Could you check a few things on this model? Use its own coordinates, in mm. A direction names the side the tool comes from. Round coordinates to 2 decimals unless told otherwise and drop trailing zeros. Write each loop counter-clockwise with the first axis right and the second up, starting at its lowest first coordinate (ties: lowest second). Pieces come first, ordered by that corner, then holes. Notation, with made-up numbers: (53, -10) -> (93, -10) arc R10 ccw to (93, 4) -> close; hole circle Ø3 at (-32.75, 79.5). An arc over 180 degrees is marked (long way). Return JSON: item names as keys, results as strings.
from build123d import *

# Parameters (mm, degrees)
SKETCH1_W           = 15
SKETCH1_H           = 10
BOSS_EXTRUDE1_DEPTH = 60
SKETCH2_W           = 15
SKETCH2_H           = 3
BOSS_EXTRUDE2_DEPTH = 10
SKETCH3_W           = 11
SKETCH3_H           = 18.791084145
CUT_EXTRUDE1_DEPTH  = 71.700070721
FILLET1_R           = 1
CUT_EXTRUDE2_DEPTH  = 72.107313267


with BuildPart() as part:
    # Sketch1 → Boss-Extrude1 (new body)
    with BuildSketch(Plane(origin=(0, 0, 0), x_dir=(1, 0, 0), z_dir=(0, 1, 0))):
        Rectangle(SKETCH1_W, SKETCH1_H)
    extrude(amount=BOSS_EXTRUDE1_DEPTH)

    # Sketch2 → Boss-Extrude2 (add)
    with BuildSketch(Plane(origin=(0, 60, 0), x_dir=(1, 0, 0), z_dir=(0, 1, 0))):
        Rectangle(SKETCH2_W, SKETCH2_H)
    extrude(amount=BOSS_EXTRUDE2_DEPTH)

    # Sketch3 → Cut-Extrude1 (cut, through all)
    with BuildSketch(Plane.XY.offset(1.5)):
        with Locations((0, 70.395542073)):
            Rectangle(SKETCH3_W, SKETCH3_H)
    extrude(amount=-CUT_EXTRUDE1_DEPTH, mode=Mode.SUBTRACT)

    # Fillet1
    fillet1_edges = [part.edges().sort_by_distance(p)[0] for p in [
        (-5.5, 70, 0),
        (5.5, 70, 0),
        (5.5, 61, 0),
        (-5.5, 61, 0),
        (-7.5, 70, 0),
        (7.5, 70, 0),
    ]]
    fillet(fillet1_edges, radius=FILLET1_R - 0.0001)  # a hair under: the kernel refuses the full size

    # Sketch4 → Cut-Extrude2 (cut, through all)
    with BuildSketch(Plane.XY.offset(5)):
        with BuildLine():
            Line((-1.5, 5), (1.5, 5))
            ThreePointArc((1.5, 5), (3.621320344, 5.878679656), (4.5, 8))
            Line((4.5, 8), (4.5, 52))
            ThreePointArc((4.5, 52), (3.621320344, 54.121320344), (1.5, 55))
            Line((1.5, 55), (-1.5, 55))
            ThreePointArc((-1.5, 55), (-3.621320344, 54.121320344), (-4.5, 52))
            Line((-4.5, 52), (-4.5, 8))
            ThreePointArc((-4.5, 8), (-3.621320344, 5.878679656), (-1.5, 5))
        make_face()
    extrude(amount=-CUT_EXTRUDE2_DEPTH, mode=Mode.SUBTRACT)


solid = part.part
1) I want a section at D-D, the plane x = -3.5. Please give me the cut outline in (y, z), and give its area (3 significant figures).
Return value:
{"outline": "(0, -5) -> (5.76, -5) -> (5.76, 5) -> (0, 5) -> close; (54.24, -5) -> (60, -5) -> (60, -1.5) -> (61, -1.5) -> (61, 1.5) -> (60, 1.5) -> (60, 5) -> (54.24, 5) -> close", "area": "118 mm²"}
2) I want a section at C-C, the plane z = -3. Please give me the cut outline in (x, y).
Return value:
{"outline": "(-7.5, 0) -> (7.5, 0) -> (7.5, 60) -> (-7.5, 60) -> close; hole (-4.5, 8) arc R3 ccw to (-1.5, 5) -> (1.5, 5) arc R3 ccw to (4.5, 8) -> (4.5, 52) arc R3 ccw to (1.5, 55) -> (-1.5, 55) arc R3 ccw to (-4.5, 52) -> close"}
3) I want a section at A-A, the plane y = 10.5. Please give me the cut outline in (x, z).
Return value:
{"outline": "(-7.5, -5) -> (-4.5, -5) -> (-4.5, 5) -> (-7.5, 5) -> close; (4.5, -5) -> (7.5, -5) -> (7.5, 5) -> (4.5, 5) -> close"}
4) If I drill on probe 1 along X at (y, z) = (37.5, 2); probe 2 along Y at (x, z) = (-1.5, -1); probe 3 along Y at (x, z) = (-7, -4.5), over which ranges is the centre line in solid material (lowest first)? Write a range as [from, to].
Return value:
{"probe 1": "[-7.5, -4.5], [4.5, 7.5]", "probe 2": "[0, 5], [55, 61]", "probe 3": "[0, 60]"}
5) For faces 1 (the face through (-7.5, 34, 0)), 2 (the face through (0, 55, 0)), 3 (the face through (0, 60, -3)), 4 (the face through (0, 60.2, 1.5)), 5 (the face through (5.5, 65, 0)), which set-ups out of +Z, -Z, +X, -X, +Y, -Y let a thin tool reach every point of the face, with its end or its side?
Return value:
{"face 1": "+Z, -Z, -X, +Y, -Y", "face 2": "+Z, -Z", "face 3": "-Z, +X, -X, +Y", "face 4": "+Z, +X, -X, +Y", "face 5": "+Z, -Z, +Y"}
6) Will these pins go through, and if not, where does the flat tip stop? pin 1 Ø0.9 at (x, z) = (-1.5, 0) entering from +Y; pin 2 Ø5 at (x, y) = (-2.5, 65) entering from +Z; pin 3 Ø1 at (x, y) = (4.5, 61) entering from +Z; pin 4 Ø1 at (x, z) = (2, -3) entering from +Y.
Return value:
{"pin 1": "y = 61", "pin 2": "through", "pin 3": "z = 1.5", "pin 4": "y = 60"}
7) Thinking about a two-plate mould opening in Y: for faces 6 (the face through (0, 60, 3)), 7 (the face through (0, 0, 0)), 8 (the face through (4.5, 30, 0)), 9 (the face through (-5.5, 65, 0)), which applies, pulls with the +Y half, pulls with the -Y half, needs draft (parallel to the pull), parting line crosses it, or undercut?
Return value:
{"face 6": "pulls with the +Y half", "face 7": "pulls with the -Y half", "face 8": "undercut", "face 9": "needs draft"}
8) I want a section at B-B, the plane x = -0.25. Please give me the cut outline in (y, z).
Return value:
{"outline": "(0, -5) -> (5, -5) -> (5, 5) -> (0, 5) -> close; (55, -5) -> (60, -5) -> (60, -1.5) -> (61, -1.5) -> (61, 1.5) -> (60, 1.5) -> (60, 5) -> (55, 5) -> close"}
